```python
from build123d import *

# Parameters (mm, degrees)
F1_DEPTH      = 12
F1_DEPTH_BACK = 28
F0_R          = 20
F2_DEPTH      = 12
F0_R_2        = 10
F3_DEPTH      = 12
F3_DEPTH_BACK = 16


with BuildPart() as f1:
    # F0 (on Front) → F1 (new body, two sides)
    with BuildSketch(Plane.XZ) as f1_sk:
        Polygon((44, -40), (-44, -40), (-44, -70), (-20, -70), (-20, -55), (20, -55), (20, -70), (44, -70), align=None)
    extrude(amount=F1_DEPTH)
    extrude(f1_sk.sketch, amount=-F1_DEPTH_BACK)

    # F0 (on Front) → F2 (join)
    with BuildSketch(Plane.XZ):
        with BuildLine():
            Line((-44, 0), (-44, -40))
            Line((-44, -40), (44, -40))
            Line((44, -40), (44, 0))
            ThreePointArc((44, 0), (31.112698, 31.112698), (0, 44))
            ThreePointArc((0, 44), (-31.112698, 31.112698), (-44, 0))
        make_face()
        Circle(F0_R, mode=Mode.SUBTRACT)
        Polygon((44, -40), (-44, -40), (-44, -70), (-20, -70), (-20, -55), (20, -55), (20, -70), (44, -70), align=None)
    extrude(amount=F2_DEPTH)

    # F0 (on Front) → F3 (join, two sides)
    with BuildSketch(Plane.XZ) as f3_sk:
        Circle(F0_R)
        Circle(F0_R_2, mode=Mode.SUBTRACT)
    extrude(amount=F3_DEPTH)
    extrude(f3_sk.sketch, amount=-F3_DEPTH_BACK)


solid = f1.part
```
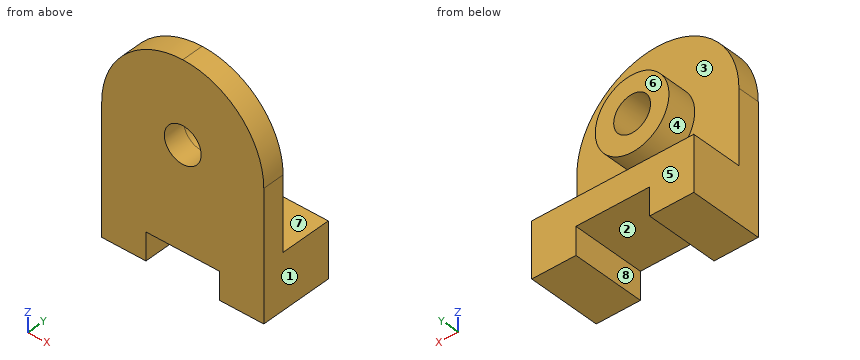
Work out the finished part from the listing and answer in its coordinate system (mm). Face numbers are marked on the shaded views. A direction names the side the tool comes from. Coordinates: 2 decimals unless noted, no trailing zeros. Write each loop counter-clockwise with the first axis right and the second up, starting at its lowest first coordinate (ties: lowest second). Pieces come first, ordered by that corner, then holes.
Q1. A cutting plane is placed at D-D, the plane x = 32. Give the vertices of the cut face in (y, z), then the cut area to 3 significant figures.
Q2. Find the intervals of material crossed by line 1 (Z direction, x = 0, y = 11); line 2 (Y direction, x = -5, z = 15.5); line 3 (Y direction, x = -21, z = 4), in increasing order.
Q3. A cutting plane is placed at B-B, the plane y = -4. Give the vertices of the cut face in (x, z), then the cut area to 3 significant figures.
Q4. Each of these flat-tipped pins is pushed along its axis until it touches: pin 1 Ø12 at (x, y) = (0.5, 4.5) entering from -Z; pin 2 Ø14 at (x, y) = (3, 15.5) entering from +Z; pin 3 Ø4 at (x, z) = (-32, 8.5) entering from +Y; pin 4 Ø18 at (x, z) = (0, 0) entering from +Y. Where does it stop, or does it pass through?
Q5. Which of the six approach directions +Z, -Z, +X, -X, +Y, -Y give full straight-line access (tool end or side, diameter ignored) to the marked faces 4, 5, 6, 7 and 8?
Q6. A cutting plane is placed at C-C, the plane y = 18.5. Give the vertices of the cut face in (x, z).
Q7. A cutting plane is placed at A-A, the plane y = 9. Give the vertices of the cut face in (x, z).
Q8. Determine the mould class of the marked faces 1, 2 and 3 for opening direction Z: released by +Z, released by -Z, zero draft, split by the parting line, or undercut.
Findings below:
1. outline: (-12, -70) - (28, -70) - (28, -40) - (0, -40) - (0, 30.2) - (-12, 30.2) - close
1. area: 2,040 mm2
2. line 1: z = -55 to -40, -20 to -10, 10 to 20
2. line 2: y = -12 to 16
2. line 3: y = -12 to 0
3. outline: (-44, -70) - (-20, -70) - (-20, -55) - (20, -55) - (20, -70) - (44, -70) - (44, 0) arc R44 ccw to (0, 44) arc R44 ccw to (-44, 0) - close; hole circle Ø20 at (0, 0)
3. area: 8,290 mm2
4. pin 1: stops at z = -55
4. pin 2: stops at z = 20
4. pin 3: stops at y = 0
4. pin 4: passes through
5. face 4: +Y
5. face 5: +Z, -Z, +X, -X, +Y
5. face 6: +Z, +X, -X, +Y
5. face 7: +X, -X, +Y
5. face 8: -Z, +Y, -Y
6. outline: (-44, -70) - (-20, -70) - (-20, -55) - (20, -55) - (20, -70) - (44, -70) - (44, -40) - (-44, -40) - close
7. outline: (-44, -70) - (-20, -70) - (-20, -55) - (20, -55) - (20, -70) - (44, -70) - (44, -40) - (-44, -40) - close; circle Ø40 at (0, 0); hole circle Ø20 at (0, 0)
8. face 1: zero draft
8. face 2: released by -Z
8. face 3: undercut
